Autodesk Inventor part; units mm, degrees
ref_plane "Work Plane1" through (0, 0, -2.75) normal (0, 0, -1) x (-1, 0, 0)
ref_plane "YZ Plane" through (0, 0, 0) normal (1, 0, 0) x (0, 1, 0)
ref_plane "XZ Plane" through (0, 0, 0) normal (0, 1, 0) x (-1, 0, 0)
sketch "Sketch1" plane through (0, 0, 0) normal (0, 1, 0) x (-1, 0, 0)
  line L0 (0, 0) -> (0, -5.5)
  line L1 (0, -5.5) -> (4.0342, -5.5)
  line L2 (4.0342, -5.5) -> (10, -3.15)
  line L3 (10, -3.15) -> (10, -2.35)
  line L4 (10, -2.35) -> (4.0342, 0)
  line L5 (4.0342, 0) -> (0, 0)
  point P0 (10, -2.75)
  dimension "d0" = 43
  dimension "d2" = 0.8
  dimension "d3" = 10
  dimension "d4" = 5.5
revolve "Revolution1" add sketch "Sketch1" angle 360 about axis through (0, 0, 0) along (0, 0, -1)
sketch "Sketch2" plane through (0, 0, -5.5) normal (0, 0, -1) x (-1, 0, 0)
  circle A0 centre (0, 0) radius 4.0342
  circle A1 centre (0, 0) radius 1
  dimension "d6" = 2
extrude "Extrusion1" cut sketch "Sketch2" against normal through all contours A1
ref_plane "Work Plane1" through (0, 0, -2.75) normal (0, 0, -1) x (-1, 0, 0)
fillet "Fillet1" radius 0.5 2 edges at (10, 0, -2.35) (10, 0, -3.15)
properties part number "pritlacne_kolecko"
For this review, take the finished solid that the model builds, in its own axes (mm). Round coordinates to 2 decimals unless told otherwise and drop trailing zeros. Loops run counter-clockwise (first coordinate to the right, second up) from the corner with the lowest first, then second, coordinate; pieces in that order, holes last.
Q1. Insertion check: pin 1 Ø4 at (x, y) = (4, 6) entering from -Z; pin 2 Ø8 at (x, y) = (7, 6.5) entering from -Z; pin 3 Ø1.5 at (y, z) = (-7.5, -3.5) entering from -X. Each pin has a flat end and moves straight along its axis. Give the tip position at first contact, or say it passes through.
Result sheet:
pin 1: stops at z = -5.04
pin 2: stops at z = -4.9
pin 3: stops at x = -7.15
Q2. Add section A-A on z = -3.7. Write out the cut boundary in (x, y), plus the area to 3 significant figures.
Result sheet:
outline: circle Ø17.21 at (0, 0); hole circle Ø2 at (0, 0)
area: 229 mm2
Q3. To check wall thickness, follow line 1 along Y through (x, z) = (0.25, -2.6); line 2 along Z through (x, y) = (-6.5, 6.25); line 3 along Y through (x, z) = (-3.5, -2.8). State the ranges of each line that lie inside material, in increasing order.
Result sheet:
line 1: y = -9.99 to -0.97, 0.97 to 9.99
line 2: z = -3.54 to -1.96
line 3: y = -9.37 to 9.37
Q4. Add section B-B on z = -1.35. Write out the cut boundary in (x, y), plus the area to 3 significant figures.
Result sheet:
outline: circle Ø14.92 at (0, 0); hole circle Ø2 at (0, 0)
area: 172 mm2
Q5. Mouldability with a two-part tool opening along X and no side actions: class faces 1 (the face through (0.95, 4.28, -5.36)), 2 (the face through (-1, -1, -5.5)), 3 (the face through (0, -1, -3)) as +X half, -X half, draft (parallel to the pull), parting line (faces both ways), or undercut.
Result sheet:
face 1: parting line
face 2: draft
face 3: undercut
